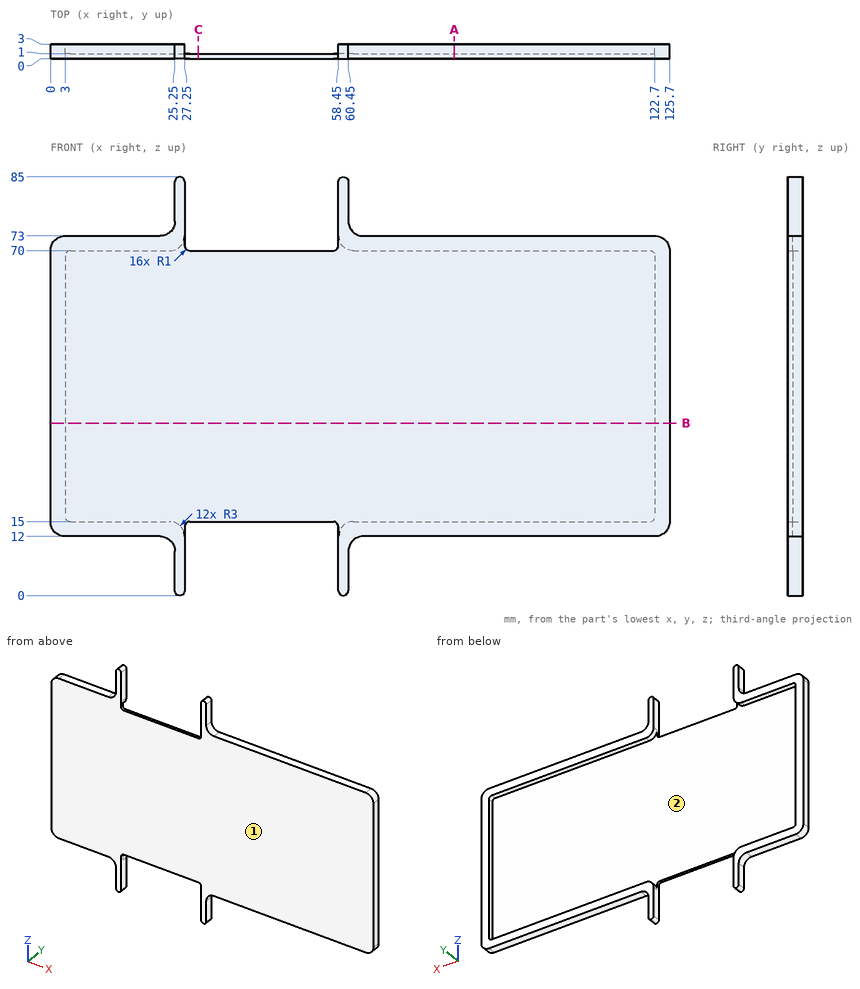
Source: three-view drawing plus pictorial views. Frame: mm from the lowest corner of the part. Round coordinates to 2 decimals unless told otherwise and drop trailing zeros. Loops run counter-clockwise (first coordinate to the right, second up) from the corner with the lowest first, then second, coordinate; pieces in that order, holes last.
Q1. Material intervals for L1, parallel to Z at x = 94, y = 1.65; L2, parallel to X at y = 1.4, z = 43.5; L3, parallel to Y at x = 38, z = 33, sorted ascending.
Q2. Pin query (flat end, axial travel): P1, Ø8, axis at x = 105.5, z = 61.5, coming from the +Y side; P2, Ø0.9, axis at y = 1.5, z = 80.5, coming from the +X side; P3, Ø1.5, axis at y = 1.5, z = 79.5, coming from the -X side. Return the tip coordinate at first contact, or that it passes through.
Q3. Pull-direction query (Z, two-part tool) for the marked faces 1 and 2; classes: released by +Z, released by -Z, zero draft, split by the parting line, or undercut.
Q4. Section C-C on x = 30. Return loops of the section in (y, z).
Q5. Section A-A on x = 82. Return loops of the section in (y, z).
Q6. Section B-B on z = 35. Return loops of the section in (x, y), plus the area to 3 significant figures.
Evaluation:
1. L1: z = 12 to 15, 70 to 73
1. L2: x = 0 to 3, 122.7 to 125.7
1. L3: y = 0 to 1
2. P1: stops at y = 1
2. P2: stops at x = 60.45
2. P3: stops at x = 25.25
3. face 1: zero draft
3. face 2: undercut
4. outline: (0, 15) - (1, 15) - (1, 70) - (0, 70) - close
5. outline: (0, 12) - (3, 12) - (3, 15) - (1, 15) - (1, 70) - (3, 70) - (3, 73) - (0, 73) - close
6. outline: (0, 0) - (125.7, 0) - (125.7, 3) - (122.7, 3) - (122.7, 1) - (3, 1) - (3, 3) - (0, 3) - close
6. area: 138 mm2
